Study the drawing (mm; zero at the part's minimum x, y, z) and answer. A direction names the side the tool comes from. Coordinates: 2 decimals unless noted, no trailing zeros. Order: outer loops, then holes, each group sorted by start corner. A loop starts at its lowest first (then second) coordinate and runs counter-clockwise, first axis right, second up. Notation, with made-up numbers: (74.25, 63.25) - (102.25, 63.25) arc R20 cw to (102.25, 76.25) - close; hole circle Ø2 at (14.25, -4). An arc over 180 degrees is marked (long way). Write item = value, one per line.
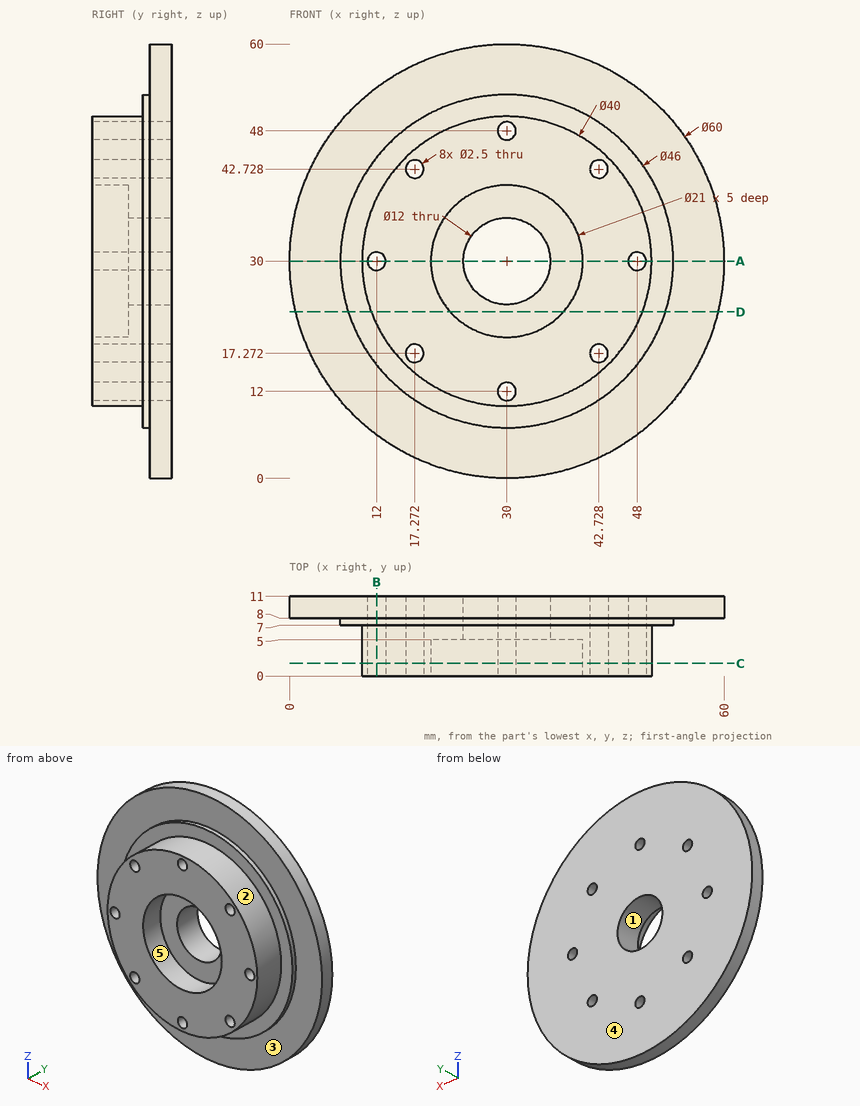
1) For the marked faces 4 and 5, determine the directions among +Z, -Z, +X, -X, +Y, -Y from which every point of the face is accessible in a straight line to the end or side of a thin tool.
Returned:
face_4 = +Z, -Z, +X, -X, +Y
face_5 = -Y
2) The part is cut by section D-D (z = 23). Determine the outline of the cut face in (x, y) (3 decimals).
Returned:
outline = (0.828, 8) - (8.091, 8) - (8.091, 7) - (11.265, 7) - (11.265, 0) - (22.174, 0) - (22.174, 5) - (37.826, 5) - (37.826, 0) - (48.735, 0) - (48.735, 7) - (51.909, 7) - (51.909, 8) - (59.172, 8) - (59.172, 11) - (0.828, 11) - close
3) Flat-ended cylindrical pins translate along their axes: pin 1 Ø3 at (x, y) = (25, 3) entering from +Z; pin 2 Ø2 at (x, z) = (11.5, 30.5) entering from -Y; pin 3 Ø1 at (y, z) = (1, 26.5) entering from +X; pin 4 Ø2 at (x, z) = (17.27, 17.27) entering from -Y. Find the tip coordinate at first contact, or state that the pin passes through.
Returned:
pin_1 = 49.69
pin_2 = 0
pin_3 = 49.77
pin_4 = through
4) The part is cut by section B-B (x = 12). Determine the outline of the cut face in (y, z), and give its area (3 significant figures).
Returned:
outline = (0, 21.28) - (7, 21.28) - (7, 15.68) - (8, 15.68) - (8, 6) - (11, 6) - (11, 28.75) - (0, 28.75) - close; (0, 31.25) - (11, 31.25) - (11, 54) - (8, 54) - (8, 44.32) - (7, 44.32) - (7, 38.72) - (0, 38.72) - close
area = 267 mm^2
5) Determine the mould class of the marked faces 1, 2 and 3 for opening direction Z: pulls with the +Z half, pulls with the -Z half, needs draft (parallel to the pull), parting line crosses it, or undercut.
Returned:
face_1 = undercut
face_2 = parting line crosses it
face_3 = needs draft
6) Straight lines are drawn through the part: line 1 along Z through (x, y) = (30, 8.55); line 2 along Z through (x, y) = (30, 1.1); line 3 along X through (y, z) = (2.25, 16.5) (1 decimal). For each, find the intervals that lie inside material, in ascending order. Write a range as from..to.
Returned:
line_1 = 0..10.75, 13.25..24, 36..46.75, 49.25..60
line_2 = 10..10.75, 13.25..19.5, 40.5..46.75, 49.25..50
line_3 = 15.2..16.3, 18.3..41.7, 43.7..44.8
7) The part is cut by section A-A (z = 30). Determine the outline of the cut face in (x, y), and give its area (3 significant figures).
Returned:
outline = (0, 8) - (7, 8) - (7, 7) - (10, 7) - (10, 0) - (10.75, 0) - (10.75, 11) - (0, 11) - close; (13.25, 0) - (19.5, 0) - (19.5, 5) - (24, 5) - (24, 11) - (13.25, 11) - close; (36, 5) - (40.5, 5) - (40.5, 0) - (46.75, 0) - (46.75, 11) - (36, 11) - close; (49.25, 0) - (50, 0) - (50, 7) - (53, 7) - (53, 8) - (60, 8) - (60, 11) - (49.25, 11) - close
area = 274 mm^2
8) The part is cut by section C-C (y = 1.75). Count the separate pieces of the cut face and the enclosed holes in it, and give its area (3 significant figures).
Returned:
separate_pieces = 1
enclosed_holes = 9
area = 871 mm^2
